Autodesk Inventor part; units mm, degrees
ref_plane "ANBAU_XY" through (14.6, -9.2, 0) normal (1, 0, 0) x (0, 0, -1)
ref_plane "ANBAU_YZ" through (14.6, -9.2, 0) normal (0, 0, -1) x (0, 1, 0)
ref_plane "ANBAU_ZX" through (14.6, -9.2, 0) normal (0, 1, 0) x (1, 0, 0)
sketch "Skizze_1" plane through (-27.55, 0, 0) normal (1, 0, 0) x (0, 0, -1)
  line L0 (-6.8, 5) -> (-6.8, 0)
  line L1 (-6.8, 0) -> (6.8, 0)
  line L2 (6.8, 0) -> (6.8, 5)
  line L3 (6.8, 5) -> (3.25, 5)
  line L4 (3.25, 5) -> (3.25, 9.8)
  line L5 (3.25, 9.8) -> (-3.25, 9.8)
  line L6 (-3.25, 9.8) -> (-3.25, 5)
  line L7 (-3.25, 5) -> (-6.8, 5)
extrude "Extrusion1" add sketch "Skizze_1" along normal blind 51.1
sketch "Skizze_2" plane through (0, 0, 0) normal (0, 0, 1) x (1, 0, 0)
  line L0 (-27.55, 7) -> (-27.55, -12.2)
  line L1 (-27.55, -12.2) -> (-23.55, -12.2)
  line L2 (-23.55, -12.2) -> (-23.55, 7)
  line L3 (-23.55, 7) -> (-27.55, 7)
extrude "Extrusion2" add sketch "Skizze_2" along normal mid plane 6
sketch "Sketch_1" plane through (0, 0, 0) normal (0, 0, 1) x (1, 0, 0)
  line L0 (14.6, -9.2) -> (-23.55, -9.2)
  line L1 (-23.55, -9.2) -> (-23.55, -6.7)
  line L2 (-23.55, -6.7) -> (9.5133, -6.7)
  line L3 (9.5133, -6.7) -> (9.5133, -1.7)
  line L4 (9.5133, -1.7) -> (14.6, -1.7)
  line L5 (14.6, -1.7) -> (14.6, -9.2)
  line L6 (14.6, -9.2) -> (-23.55, -9.2)
revolve "Revolution1" add sketch "Sketch_1" angle 360 about axis through (14.6, -9.2, 0) along (1, 0, 0)
sketch "Sketch_3" plane through (19.25, 0, 0) normal (1, 0, 0) x (0, 0, -1)
  line L0 (0, 9.8) -> (0, 0.6401)
  line L1 (0, 0.6401) -> (-1.2295, 1.35)
  line L2 (-1.2295, 1.35) -> (-1.2295, 8.2295)
  line L3 (-1.2295, 8.2295) -> (-1.5, 8.5)
  line L4 (-1.5, 8.5) -> (-2.5, 8.5)
  line L5 (-2.5, 8.5) -> (-2.5, 9.8)
  line L6 (-2.5, 9.8) -> (0, 9.8)
  line L7 (0, 9.8) -> (0, 0.6401)
revolve "Revolution2" cut sketch "Sketch_3" angle 360 about axis through (19.25, 9.8, 0) along (0, 1, 0)
thread "Thread1"
pattern_linear "Rectangular Pattern1" count 3 spacing 8 along (-1, 0, 0) of "Revolution2"
ref_plane "ANBAU_XY" through (14.6, -9.2, 0) normal (1, 0, 0) x (0, 0, -1)
ref_plane "ANBAU_YZ" through (14.6, -9.2, 0) normal (0, 0, -1) x (0, 1, 0)
ref_plane "ANBAU_ZX" through (14.6, -9.2, 0) normal (0, 1, 0) x (1, 0, 0)
ref_plane "SCHRAUBE_1_XY" through (19.25, 8.5, 0) normal (0, 1, 0) x (1, 0, 0)
ref_plane "SCHRAUBE_1_YZ" through (19.25, 8.5, 0) normal (1, 0, 0) x (0, 0, -1)
ref_plane "SCHRAUBE_1_ZX" through (19.25, 8.5, 0) normal (0, 0, -1) x (0, 1, 0)
ref_plane "SCHRAUBE_2_XY" through (11.25, 8.5, 0) normal (0, 1, 0) x (1, 0, 0)
ref_plane "SCHRAUBE_2_YZ" through (11.25, 8.5, 0) normal (1, 0, 0) x (0, 0, -1)
ref_plane "SCHRAUBE_2_ZX" through (11.25, 8.5, 0) normal (0, 0, -1) x (0, 1, 0)
ref_plane "SCHRAUBE_3_XY" through (3.25, 8.5, 0) normal (0, 1, 0) x (1, 0, 0)
ref_plane "SCHRAUBE_3_YZ" through (3.25, 8.5, 0) normal (1, 0, 0) x (0, 0, -1)
ref_plane "SCHRAUBE_3_ZX" through (3.25, 8.5, 0) normal (0, 0, -1) x (0, 1, 0)
ref_plane "ZBHJAW1_XY" through (19.25, 8.5, 0) normal (0, -1, 0) x (1, 0, 0)
ref_plane "ZBHJAW1_YZ" through (19.25, 8.5, 0) normal (1, 0, 0) x (0, 0, 1)
ref_plane "ZBHJAW1_ZX" through (19.25, 8.5, 0) normal (0, 0, 1) x (0, -1, 0)
ref_plane "ZBHJAW2_XY" through (3.25, 8.5, 0) normal (0, -1, 0) x (1, 0, 0)
ref_plane "ZBHJAW2_YZ" through (3.25, 8.5, 0) normal (1, 0, 0) x (0, 0, 1)
ref_plane "ZBHJAW2_ZX" through (3.25, 8.5, 0) normal (0, 0, 1) x (0, -1, 0)
properties part number "3361610 HGPL-BAC-14-20---(J)"
Work out the finished part from the listing and answer in its coordinate system (mm). A direction names the side the tool comes from. Give positions to 0.01 mm unless a question says otherwise; leave off trailing zeros. Write each loop counter-clockwise with the first axis right and the second up, starting at its lowest first coordinate (ties: lowest second). Pieces come first, ordered by that corner, then holes. Notation, with made-up numbers: M 63.5,-25.5 L 101.5,-25.5 A25 ccw 101.5,8.5 Z; hole C -12,18 d4. An arc over 180 degrees is marked long. Answer as CSV lines item,"result".
Q1. A cutting plane is placed at C-C on y = -9.2. Write down the section's boundary in (x, z).
A:
outline,"M -27.55,-3 L -23.55,-3 L -23.55,-2.5 L 9.51,-2.5 L 9.51,-7.5 L 14.6,-7.5 L 14.6,7.5 L 9.51,7.5 L 9.51,2.5 L -23.55,2.5 L -23.55,3 L -27.55,3 Z"
Q2. A cutting plane is placed at D-D on y = -2.5. Write down the section's boundary in (x, z).
A:
outline,"M -27.55,-3 L -23.55,-3 L -23.55,3 L -27.55,3 Z; M 9.51,-3.37 L 14.6,-3.37 L 14.6,3.37 L 9.51,3.37 Z"
Q3. A cutting plane is placed at A-A on x = -15. Write down the section's boundary in (y, z), plus the area to 3 significant figures.
A:
outline,"C -9.2,0 d5; M 0,-6.8 L 5,-6.8 L 5,-3.25 L 9.8,-3.25 L 9.8,3.25 L 5,3.25 L 5,6.8 L 0,6.8 Z"
area,"119 mm²"
Q4. The mould has two halves that part along Y. Classify faces 5 (the cylindrical face through (12.092, -16.693, 0.33)), 6 (the conical face through (3.042, 0.763, -0.046)), 7 (the cylindrical face through (8.8, 9.2, -0.5)): +Y half, -Y half, draft (parallel to the pull), parting line (faces both ways), or undercut.
A:
face 5,"undercut"
face 6,"+Y half"
face 7,"draft"
Q5. Find the intervals of material crossed by probe 1 along X at (y, z) = (8.8, 0); probe 2 along Y at (x, z) = (-20, 4.5); probe 3 along Z at (x, y) = (15.5, 6.25), in increasing order. Write a range as [from, to].
A:
probe 1,"x = [-27.55, 0.75], [5.75, 8.75], [13.75, 16.75], [21.75, 23.55]"
probe 2,"y = [0, 5]"
probe 3,"z = [-3.25, 3.25]"
Q6. A cutting plane is placed at B-B on z = 5.75. Write down the section's boundary in (x, y), plus the area to 3 significant figures.
A:
outline,"M -27.55,0 L 23.55,0 L 23.55,5 L -27.55,5 Z; M 9.51,-14.02 L 14.6,-14.02 L 14.6,-4.38 L 9.51,-4.38 Z"
area,"304 mm²"
Q7. A tool of negligible diameter and unlimited length cuts with its end or side. For faces 1 (the flat face through (-26, -6, -3)), 2 (the cylindrical face through (18.05, 4.84, -0.27)), 3 (the flat face through (-2, 5, 5)), 4 (the flat face through (-26, -12.2, 0)), from which of +Z, -Z, +X, -X, +Y, -Y can it reach the whole face along a straight path? Write none if from no direction.
A:
face 1,"-Z, -X, -Y"
face 2,"+Y"
face 3,"+Z, +X, -X, +Y"
face 4,"+Z, -Z, -X, -Y"
Q8. Given P1, Ø4, axis at x = 2, z = 5.5, coming from the +Y side; P2, Ø3, axis at x = -10, z = -4.5, coming from the +Y side; P3, Ø5.5, axis at x = 7, y = 8.5, coming from the -Z side; P4, Ø5.5, axis at x = 3, y = 2, coming from the +Z side, each flat-ended and moving along its own axis, determine where each tip first touches the part or whether it passes through.
A:
P1,"stops at y = 5"
P2,"stops at y = 9.8"
P3,"stops at z = -3.25"
P4,"stops at z = 6.8"
